```python
from build123d import *

# Parameters (mm, degrees)
F1_DEPTH = 3.302
F2_W     = 190.5
F2_H     = 284.48
F3_DEPTH = 1.016


with BuildPart() as f1:
    # F0 (on Top) → F1 (new body)
    with BuildSketch(Plane.XY):
        with BuildLine():
            Line((91.44, 146.05), (-91.44, 146.05))
            ThreePointArc((-91.44, 146.05), (-94.134077, 144.934077), (-95.25, 142.24))
            Line((-95.25, 142.24), (-95.25, -142.24))
            ThreePointArc((-95.25, -142.24), (-94.134077, -144.934077), (-91.44, -146.05))
            Line((-91.44, -146.05), (91.44, -146.05))
            ThreePointArc((91.44, -146.05), (94.134077, -144.934077), (95.25, -142.24))
            Line((95.25, -142.24), (95.25, 142.24))
            ThreePointArc((95.25, 142.24), (94.134077, 144.934077), (91.44, 146.05))
        make_face()
    extrude(amount=F1_DEPTH)

    # F2 (on face) → F3 (cut)
    with BuildSketch(Plane.XY.offset(3.302)):
        Rectangle(F2_W, F2_H)
    extrude(amount=-F3_DEPTH, mode=Mode.SUBTRACT)


solid = f1.part
```
The listing builds one solid part. Answer for the finished solid, in the listing's coordinates (mm). Give positions to 0.01 mm unless a question says otherwise; leave off trailing zeros. Order: outer loops, then holes, each group sorted by start corner. A loop starts at its lowest first (then second) coordinate and runs counter-clockwise, first axis right, second up.
1) Consider line 1 along Y through (x, z) = (-1.5, 2.35); line 2 along Z through (x, y) = (-56, 32.5). Determine where each line is inside the solid, lowest interval first.
Reported:
line 1: y = -146.05 to -142.24, 142.24 to 146.05
line 2: z = 0 to 2.29
2) Find section B-B on y = 37. Write down the section's boundary in (x, z).
Reported:
outline: (-95.25, 0) - (95.25, 0) - (95.25, 2.29) - (-95.25, 2.29) - close
3) Find section A-A on x = -6. Write down the section's boundary in (y, z).
Reported:
outline: (-146.05, 0) - (146.05, 0) - (146.05, 3.3) - (142.24, 3.3) - (142.24, 2.29) - (-142.24, 2.29) - (-142.24, 3.3) - (-146.05, 3.3) - close
4) Determine the mould class of faces 1 (the face through (-1, 2, 0)), 2 (the face through (-1, 2, 2.286)) for opening direction Y: pulls with the +Y half, pulls with the -Y half, needs draft (parallel to the pull), parting line crosses it, or undercut.
Reported:
face 1: needs draft
face 2: undercut
5) Given P1, Ø4, axis at x = -68, y = -26, coming from the +Z side, flat-ended and moving along its own axis, determine where the tip first touches the part or whether it passes through.
Reported:
P1: stops at z = 2.29
